Geometry check sheet. Reference: the model listing, model coordinates, mm. Face numbers are marked on the shaded views. Give positions to 0.01 mm unless a question says otherwise; leave off trailing zeros. Order: outer loops, then holes, each group sorted by start corner. A loop starts at its lowest first (then second) coordinate and runs counter-clockwise, first axis right, second up. Notation, with made-up numbers: M 64.25,82.5 L 109.25,82.5 A7 cw 109.25,87.5 Z; hole C 23,7 d8. An arc over 180 degrees is marked long. Use CSV: the item, a comma, the result in double quotes. Start each with the question number.
from build123d import *

# Parameters (mm, degrees)
F0_R     = 2.25
F0_R_2   = 3.75
F0_R_3   = 11
F1_DEPTH = 12


with BuildPart() as f1:
    # F0 (on Front) → F1 (new body)
    with BuildSketch(Plane.XZ):
        with BuildLine():
            Line((0, 40), (0, 0))
            Line((0, 0), (87, 0))
            Line((87, 0), (87, 40))
            Line((87, 40), (64.238746, 79.07909))
            ThreePointArc((64.238746, 79.07909), (43.5, 91), (22.761254, 79.07909))
            Line((22.761254, 79.07909), (0, 40))
        make_face()
        with Locations((12, 5)):
            Circle(F0_R, mode=Mode.SUBTRACT)
        with Locations((8, 34)):
            Circle(F0_R_2, mode=Mode.SUBTRACT)
        with Locations((75, 5)):
            Circle(F0_R, mode=Mode.SUBTRACT)
        with Locations((79, 34)):
            Circle(F0_R_2, mode=Mode.SUBTRACT)
        with Locations((43.5, 67)):
            Circle(F0_R_3, mode=Mode.SUBTRACT)
    extrude(amount=F1_DEPTH)


solid = f1.part
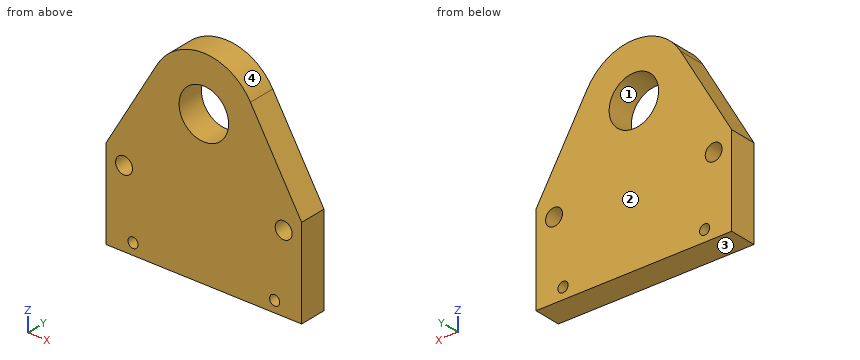
(1) Sectioned sample at D-D on z = 67. Record the cut outline in (x, y).
(2) Draft check along Z on the marked faces 1, 2, 3 and 4. Enter one of: +Z half, -Z half, draft (parallel to the pull), parting line (faces both ways), or undercut.
(3) Sectioned sample at B-B on x = 43.5. Record the cut outline in (y, z).
(4) Sectioned sample at C-C on y = -2.75. Record the cut outline in (x, z).
(5) Thickness scan on line 1 (Z direction, x = 10, y = -10); line 2 (Z direction, x = 76, y = -5.75); line 3 (X direction, y = -6, z = 36). Record the ranges inside material, lowest first.
(6) Sectioned sample at A-A on z = 5. Record the cut outline in (x, y), then the cut area to 3 significant figures.
Responses:
1,outline,"M 15.73,-12 L 32.5,-12 L 32.5,0 L 15.73,0 Z; M 54.5,-12 L 71.27,-12 L 71.27,0 L 54.5,0 Z"
2,face 1,"undercut"
2,face 2,"draft"
2,face 3,"-Z half"
2,face 4,"+Z half"
3,outline,"M -12,0 L 0,0 L 0,56 L -12,56 Z; M -12,78 L 0,78 L 0,91 L -12,91 Z"
4,outline,"M 0,0 L 87,0 L 87,40 L 64.24,79.08 A24 ccw 22.76,79.08 L 0,40 Z; hole C 8,34 d7.5; hole C 12,5 d4.5; hole C 43.5,67 d22; hole C 75,5 d4.5; hole C 79,34 d7.5"
5,line 1,"0 to 3.97, 6.03 to 30.83, 37.17 to 57.17"
5,line 2,"0 to 2.98, 7.02 to 31.75, 36.25 to 58.89"
5,line 3,"0 to 4.83, 11.17 to 75.83, 82.17 to 87"
6,outline,"M 0,-12 L 9.75,-12 L 9.75,0 L 0,0 Z; M 14.25,-12 L 72.75,-12 L 72.75,0 L 14.25,0 Z; M 77.25,-12 L 87,-12 L 87,0 L 77.25,0 Z"
6,area,"936 mm2"
